The model under review builds one solid part; all positions refer to its coordinate system, in mm. A direction names the side the tool comes from. Give positions to 0.01 mm unless a question says otherwise; leave off trailing zeros. Order: outer loops, then holes, each group sorted by start corner. A loop starts at its lowest first (then second) coordinate and runs counter-clockwise, first axis right, second up. Notation, with made-up numbers: (47.25, -30) - (104.25, -30) arc R27 ccw to (104.25, -5) - close; hole circle Ø4 at (3, 38). An arc over 180 degrees is marked (long way). Write item = value, one per line. Start each with the question number.
1. We need section B-B, the plane x = 3.5. Give the boundary of the cut face in (y, z).
2. Machinability: for faces 5 (the cylindrical face through (44.704, 2.535, 44.603)), 6 (the flat face through (59, 2, 8.039)), 7 (the cylindrical face through (36.307, 1.232, 19.893)), 8 (the flat face through (8.27, 2, 31)), which of the approach directions +Z, -Z, +X, -X, +Y, -Y give a long, thin tool a straight path to every point of the face, cutting with its end or side? Answer none if there is none.
3. We need section A-A, the plane z = 47. Give the boundary of the cut face in (x, y), and give its area (3 significant figures).
4. For P1, Ø1, axis at y = 2.5, z = 39.5, coming from the -X side; P2, Ø4, axis at x = 46.27, z = 15.04, coming from the -Y side; P3, Ø5, axis at x = 14.5, z = 11.5, coming from the -Y side; P4, Ø1.5, axis at y = 3.5, z = 34.5, coming from the +X side, all flat-tipped, find the tip position at first contact; note any pin that passes through.
5. Wall thickness on probe 1 along Z at (x, y) = (58, 3.2); probe 2 along Z at (x, y) = (46.5, 0.8); probe 3 along X at (y, z) = (0.8, 45): over which ranges is each line inside the solid? List them lowest first.
6. We need section D-D, the plane y = 1.1. State how many separate pieces and enclosed holes the cut face has, and give its area (3 significant figures).
7. We need section C-C, the plane z = 28.5. Give the boundary of the cut face in (x, y).
8. Mouldability with a two-part tool opening along Z and no side actions: class faces 1 (the flat face through (31, 2, -8.961)), 2 (the flat face through (36, 2.5, 31)), 3 (the cylindrical face through (2.222, 2.535, -3.505)), 4 (the flat face through (65.77, 2, 0)) as pulls with the +Z half, pulls with the -Z half, needs draft (parallel to the pull), parting line crosses it, or undercut.
Autodesk Inventor part; units mm, degrees
ref_plane "YZ Plane" through (0, 0, 0) normal (1, 0, 0) x (0, 1, 0)
ref_plane "XZ Plane" through (0, 0, 0) normal (0, 1, 0) x (-1, 0, 0)
ref_plane "XY Plane" through (0, 0, 0) normal (0, 0, 1) x (1, 0, 0)
sketch "Skizze1" plane through (0, 0, 0) normal (0, 1, 0) x (-1, 0, 0)
  line L0 (4.2298, 8.039) -> (-65.7702, 8.039)
  line L1 (-65.7702, 8.039) -> (-65.7702, -8.961)
  line L2 (-65.7702, -8.961) -> (4.2298, -8.961)
  line L3 (4.2298, -8.961) -> (4.2298, 8.039)
  line L4 (-8.2702, 8.039) -> (-53.2702, 8.039)
  line L5 (-53.2702, 8.039) -> (-53.2702, 53.039)
  line L6 (-53.2702, 53.039) -> (-8.2702, 53.039)
  line L7 (-8.2702, 53.039) -> (-8.2702, 8.039)
  point P0 (0, 0)
  dimension "d0" = 70
  dimension "d1" = 17
  dimension "d2" = 45
  dimension "d3" = 45
  dimension "d4" = 12.5
extrude "Extrusion1" add sketch "Skizze1" along normal blind 5
sketch "Skizze2" plane through (0, 5, 0) normal (0, 1, 0) x (1, 0, 0)
  point P0 (0, 0)
sketch "Skizze3" plane through (0, 5, 0) normal (0, 1, 0) x (1, 0, 0)
  circle A0 centre (0, 0) radius 2.1
  circle A1 centre (12.7702, 2.086) radius 2.1
  circle A2 centre (48.7702, 2.086) radius 2.1
  circle A3 centre (57.7702, 2.086) radius 2.1
  line L0 (65.7702, -8.039) -> (65.7702, 8.961)
  line L1 (65.7702, 8.961) -> (-4.2298, 8.961)
  line L2 (-4.2298, 8.961) -> (-4.2298, -8.039)
  dimension "d7" = 4.2
  dimension "d8" = 4.2
  dimension "d9" = 4.2
  dimension "d10" = 4.2
  dimension "d11" = 8
  dimension "d12" = 17
  dimension "d13" = 6.875
  dimension "d14" = 6.875
  dimension "d15" = 6.875
  dimension "d16" = 8.961
  dimension "d17" = 17
sketch "Skizze4" plane through (0, 5, 0) normal (0, 1, 0) x (1, 0, 0)
  circle A0 centre (3.7702, 2.086) radius 2.1
  line L0 (65.7702, 8.961) -> (-4.2298, 8.961)
  line L1 (-4.2298, 8.961) -> (-4.2298, -8.039)
  point P0 (0, 0)
  dimension "d18" = 4.2
  dimension "d19" = 6.875
  dimension "d20" = 8
extrude "Extrusion2" cut sketch "Skizze4" against normal blind 20
extrude "Extrusion3" cut sketch "Skizze3" against normal blind 20 contours A1 | A2 | A3
sketch "Skizze5" plane through (0, 5, 0) normal (0, 1, 0) x (1, 0, 0)
  line L0 (9.6202, -51.689) -> (51.9202, -51.689)
  line L1 (51.9202, -51.689) -> (51.9202, -9.389)
  line L2 (51.9202, -9.389) -> (9.6202, -9.389)
  line L3 (9.6202, -9.389) -> (9.6202, -51.689)
  line L4 (8.2702, -8.039) -> (8.2702, -53.039)
  line L5 (8.2702, -53.039) -> (53.2702, -53.039)
  line L6 (15.2702, -46.039) -> (46.2702, -46.039)
  line L7 (46.2702, -46.039) -> (46.2702, -15.039)
  line L8 (46.2702, -15.039) -> (15.2702, -15.039)
  line L9 (15.2702, -15.039) -> (15.2702, -46.039)
  circle A0 centre (15.2702, -46.039) radius 2.125
  circle A1 centre (15.2702, -15.039) radius 2.125
  circle A2 centre (46.2702, -46.039) radius 2.125
  circle A3 centre (46.2702, -15.039) radius 2.125
  line L10 (15.2702, -46.039) -> (46.2702, -15.039)
  line L11 (46.2702, -46.039) -> (15.2702, -15.039)
  circle A4 centre (30.7702, -30.539) radius 4.25
  point P0 (0, 0)
  dimension "d25" = 42.3
  dimension "d26" = 42.3
  dimension "d27" = 1.35
  dimension "d28" = 1.35
  dimension "d29" = 31
  dimension "d30" = 31
  dimension "d31" = 5.65
  dimension "d32" = 5.65
  dimension "d33" = 4.25
  dimension "d34" = 4.25
  dimension "d35" = 4.25
  dimension "d36" = 4.25
  dimension "d37" = 8.5
extrude "Extrusion4" cut sketch "Skizze5" against normal blind 20 contours L10 A0 L6 | L6 A0 L9 | L9 A0 L10 | A2 L11 L6 | L6 L7 A2 | A1 L8 L9 | L9 L11 A1 | A4 L11 L10 | L10 L11 A4 | L11 A2 L7 | L8 A1 L11 | L11 A4 L10 | L10 A4 L11 | A3 L7 L8 | L8 L10 A3 | A3 L10 L7
sketch "Skizze6" plane through (0, 0, 0) normal (0, -1, 0) x (1, 0, 0)
  circle A0 centre (46.2702, 46.039) radius 2.125
  circle A1 centre (15.2702, 15.039) radius 2.125
  line L0 (46.2702, 46.039) -> (15.2702, 46.039)
  line L1 (15.2702, 46.039) -> (15.2702, 15.039)
  line L2 (15.2702, 15.039) -> (46.2702, 15.039)
  line L3 (46.2702, 15.039) -> (46.2702, 46.039)
  line L4 (15.2702, 15.039) -> (46.2702, 46.039)
  line L5 (46.2702, 15.039) -> (15.2702, 46.039)
  circle A2 centre (30.7702, 30.539) radius 12
  point P0 (0, 0)
  dimension "d40" = 24
extrude "Extrusion5" cut sketch "Skizze6" against normal blind 2.5 contours A2 L5 L4 | L4 L5 A2 | L5 L4 A2 | A2 L4 L5
properties part number "YAchseMotorteil"
Model answer:
q1.outline = (0, -8.96) - (5, -8.96) - (5, -4.17) - (0, -4.17) - close; (0, 0) - (5, 0) - (5, 8.04) - (0, 8.04) - close
q2.face_5 = +Y, -Y
q2.face_6 = +Z, +X, +Y, -Y
q2.face_7 = -Y
q2.face_8 = +Z, -X, +Y, -Y
q3.outline = (8.27, 0) - (13.37, 0) - (13.37, 5) - (8.27, 5) - close; (17.17, 0) - (44.37, 0) - (44.37, 5) - (17.17, 5) - close; (48.17, 0) - (53.27, 0) - (53.27, 5) - (48.17, 5) - close
q3.area = 187 mm2
q4.P1 = 8.27
q4.P2 = through
q4.P3 = 0
q4.P4 = 53.27
q5.probe_1 = -8.96 to -4.17, 0 to 8.04
q5.probe_2 = -8.96 to 12.93, 17.15 to 43.93, 48.15 to 53.04
q5.probe_3 = 8.27 to 13.42, 17.12 to 44.42, 48.12 to 53.27
q6.separate_pieces = 1
q6.enclosed_holes = 9
q6.area = 2,650 mm2
q7.outline = (8.27, 0) - (18.94, 0) - (18.94, 2.5) - (27.04, 2.5) - (27.04, 5) - (8.27, 5) - close; (34.5, 2.5) - (42.6, 2.5) - (42.6, 0) - (53.27, 0) - (53.27, 5) - (34.5, 5) - close
q8.face_1 = pulls with the -Z half
q8.face_2 = undercut
q8.face_3 = undercut
q8.face_4 = needs draft
